from build123d import *

# Parameters (mm, degrees)
SKETCH_2_R                       = 1.75
EXTRUDE_1_DEPTH                  = 3
CUT_EXTRUDE_1_REACH              = 62.067
SKETCH_3_R                       = 13.5
EXTRUDE_START                    = -3
SKETCH_4_R                       = 3.75
SKETCH_4_R_2                     = 1.75
EXTRUDE_2_DEPTH                  = 3
FILLET_1_R                       = 1
PATTERN_CIRCULAR_1_COUNT         = 6
FILLET_1_OF_PATTERN_CIRCULAR_1_R = 1


with BuildPart() as part:
    # Sketch 2 → Extrude 1 (new body)
    # profile 1 of 5: a face of its own
    with BuildSketch(Plane(origin=(0, 0, 0), x_dir=(1, 0, 0), z_dir=(0, 1, 0))):
        with BuildLine():
            ThreePointArc((51.423130363, -9.332273137), (45.983390632, 4.986611908), (32.408442676, 12.08182334))
            ThreePointArc((32.408442676, 12.08182334), (21.996560251, 10.749395349), (13.44709691, 4.659293825))
            ThreePointArc((13.44709691, 4.659293825), (14.101694562, 1.915015852), (13.429705605, -0.82505541))
            ThreePointArc((13.429705605, -0.82505541), (11.883124263, -4.954311801), (11.357646636, -9.332273137))
            ThreePointArc((11.357646636, -9.332273137), (10.786787874, -12.531492943), (9.144672071, -15.335836498))
            ThreePointArc((9.144672071, -15.335836498), (13.315451151, -23.167946482), (20.286858748, -28.657647844))
            ThreePointArc((20.286858748, -28.657647844), (41.230232488, -27.655329089), (51.423130363, -9.332273137))
        make_face()
        with Locations(Location((16.434252877, -17.082273137, 0), (0, 0, 270))):
            Circle(SKETCH_2_R, mode=Mode.SUBTRACT)
        with Locations(Location((29.857646636, -24.832273137, 0), (0, 0, 270))):
            Circle(SKETCH_2_R, mode=Mode.SUBTRACT)
        with Locations(Location((43.281040395, -17.082273137, 0), (0, 0, 270))):
            Circle(SKETCH_2_R, mode=Mode.SUBTRACT)
        with Locations(Location((16.434252877, -1.582273137, 0), (0, 0, 270))):
            Circle(SKETCH_2_R, mode=Mode.SUBTRACT)
        with Locations(Location((43.281040395, -1.582273137, 0), (0, 0, 270))):
            Circle(SKETCH_2_R, mode=Mode.SUBTRACT)
        with Locations(Location((29.857646636, 6.167726863, 0), (0, 0, 270))):
            Circle(SKETCH_2_R, mode=Mode.SUBTRACT)
    # profile 2 of 5: a face of its own
    with BuildSketch(Plane(origin=(0, 0, 0), x_dir=(1, 0, 0), z_dir=(0, 1, 0))):
        with BuildLine():
            ThreePointArc((13.429705605, -0.82505541), (14.101694562, 1.915015852), (13.44709691, 4.659293825))
            ThreePointArc((13.44709691, 4.659293825), (8.774707488, -4.795780521), (9.144672071, -15.335836498))
            ThreePointArc((9.144672071, -15.335836498), (10.786787874, -12.531492943), (11.357646636, -9.332273137))
            ThreePointArc((11.357646636, -9.332273137), (11.883124263, -4.954311801), (13.429705605, -0.82505541))
        make_face()
    # profile 3 of 5: a face of its own
    with BuildSketch(Plane(origin=(0, 0, 0), x_dir=(1, 0, 0), z_dir=(0, 1, 0))):
        with BuildLine():
            ThreePointArc((-3.33566455, 16.339576043), (-3.689884424, 16.371156277), (-4.04535307, 16.381695363))
            Line((-4.04535307, 16.381695363), (-7.902002826, 16.381695363))
            ThreePointArc((-7.902002826, 16.381695363), (-11.154056436, 15.423931704), (-13.367877124, 12.856411137))
            ThreePointArc((-13.367877124, 12.856411137), (-13.731255095, 12.088797564), (-14.12049634, 11.333969504))
            ThreePointArc((-14.12049634, 11.333969504), (-14.757788596, 7.532855597), (-12.951275808, 4.128282218))
            ThreePointArc((-12.951275808, 4.128282218), (-8.656551428, -2.002025351), (-7.142353364, -9.332273137))
            ThreePointArc((-7.142353364, -9.332273137), (-5.751591288, -14.210272651), (-1.997514606, -17.62143179))
            ThreePointArc((-1.997514606, -17.62143179), (3.966394433, -18.393595151), (9.144672071, -15.335836498))
            ThreePointArc((9.144672071, -15.335836498), (8.774707488, -4.795780521), (13.44709691, 4.659293825))
            ThreePointArc((13.44709691, 4.659293825), (11.883867195, 6.59187417), (9.671521613, 7.725047131))
            ThreePointArc((9.671521613, 7.725047131), (4.722427963, 10.031982506), (0.837283213, 13.868794863))
            ThreePointArc((0.837283213, 13.868794863), (-0.988440561, 15.544571103), (-3.33566455, 16.339576043))
        make_face()
        with Locations(Location((2.107646636, -14.332273137, 0), (0, 0, 270))):
            Circle(SKETCH_2_R, mode=Mode.SUBTRACT)
        with Locations(Location((-2.222480383, -6.832273137, 0), (0, 0, 270))):
            Circle(SKETCH_2_R, mode=Mode.SUBTRACT)
        with Locations(Location((6.437773655, -6.832273137, 0), (0, 0, 270))):
            Circle(SKETCH_2_R, mode=Mode.SUBTRACT)
        with Locations(Location((8.10172473, 1.934042232, 0), (0, 0, 270))):
            Circle(SKETCH_2_R, mode=Mode.SUBTRACT)
        with Locations(Location((-7.902002826, 10.381695363, 0), (0, 0, 270))):
            Circle(SKETCH_2_R, mode=Mode.SUBTRACT)
    # profile 4 of 5: a face of its own
    with BuildSketch(Plane(origin=(0, 0, 0), x_dir=(1, 0, 0), z_dir=(0, 1, 0))):
        with BuildLine():
            Line((32.408442676, 12.08182334), (-3.33566455, 16.339576043))
            ThreePointArc((-3.33566455, 16.339576043), (-0.988440561, 15.544571103), (0.837283213, 13.868794863))
            ThreePointArc((0.837283213, 13.868794863), (4.722427963, 10.031982506), (9.671521613, 7.725047131))
            ThreePointArc((9.671521613, 7.725047131), (11.883867195, 6.59187417), (13.44709691, 4.659293825))
            ThreePointArc((13.44709691, 4.659293825), (21.996560251, 10.749395349), (32.408442676, 12.08182334))
        make_face()
    # profile 5 of 5: a face of its own
    with BuildSketch(Plane(origin=(0, 0, 0), x_dir=(1, 0, 0), z_dir=(0, 1, 0))):
        with BuildLine():
            Line((-1.997514606, -17.62143179), (20.286858748, -28.657647844))
            ThreePointArc((20.286858748, -28.657647844), (13.315451151, -23.167946482), (9.144672071, -15.335836498))
            ThreePointArc((9.144672071, -15.335836498), (3.966394433, -18.393595151), (-1.997514606, -17.62143179))
        make_face()
    extrude(amount=EXTRUDE_1_DEPTH)

    # Sketch 3 → Cut-Extrude 1 (cut, up to next)
    with BuildSketch(Plane(origin=(0, 3, 0), x_dir=(1, 0, 0), z_dir=(0, 1, 0)), mode=Mode.PRIVATE) as cut_extrude_1_sk1:
        with Locations(Location((29.857646636, -9.332273137, 0), (0, 0, 270))):
            Circle(SKETCH_3_R)
    cut_extrude_1_tool1 = extrude(cut_extrude_1_sk1.sketch, amount=-CUT_EXTRUDE_1_REACH, mode=Mode.PRIVATE) & part.part
    add(cut_extrude_1_tool1.solids().sort_by_distance((29.857647, 3, 9.332273))[0], mode=Mode.SUBTRACT)

    # Sketch 4 → Extrude 2 (add)
    with BuildSketch(Plane(origin=(0, 3, 0), x_dir=(1, 0, 0), z_dir=(0, 1, 0)).offset(EXTRUDE_START)):
        with Locations((29.857646636, 6.167726863)):
            Circle(SKETCH_4_R)
        with Locations(Location((29.857646636, 6.167726863, 0), (0, 0, 270))):
            Circle(SKETCH_4_R_2, mode=Mode.SUBTRACT)
    extrude_2 = extrude(amount=EXTRUDE_2_DEPTH)

    # Fillet 1
    fillet_1_edges = [part.edges().sort_by_distance(p)[0] for p in [
        (32.800222011, 1.5, -3.843130088),
        (26.915071261, 1.5, -3.843130088),
    ]]
    fillet(fillet_1_edges, radius=FILLET_1_R)

    # Pattern Circular 1: Extrude 2 ×6 about axis
    pattern_circular_1_axis = Axis((29.857646636, 0, 9.332273137), (0, 1, 0))
    for i in range(1, PATTERN_CIRCULAR_1_COUNT):
        add(extrude_2.rotate(pattern_circular_1_axis, i * 360 / PATTERN_CIRCULAR_1_COUNT))

    # Fillet 1 of Pattern Circular 1
    fillet_1_of_pattern_circular_1_edges = [part.edges().sort_by_distance(p)[0] for p in [
        (19.918700425, 1.5, 0.196226497),
        (16.97612505, 1.5, 5.292916552),
        (16.97612505, 1.5, 13.371629723),
        (19.918700425, 1.5, 18.468319778),
        (26.915071261, 1.5, 22.507676363),
        (32.800222011, 1.5, 22.507676363),
        (39.796592847, 1.5, 18.468319778),
        (42.739168222, 1.5, 13.371629723),
        (42.739168222, 1.5, 5.292916552),
        (39.796592847, 1.5, 0.196226497),
    ]]
    fillet(fillet_1_of_pattern_circular_1_edges, radius=FILLET_1_OF_PATTERN_CIRCULAR_1_R)


solid = part.part
Work out the finished part from the listing and answer in its coordinate system (mm). A direction names the side the tool comes from. Coordinates: 2 decimals unless noted, no trailing zeros. Write each loop counter-clockwise with the first axis right and the second up, starting at its lowest first coordinate (ties: lowest second). Pieces come first, ordered by that corner, then holes. Notation, with made-up numbers: M 79,30 L 111,30 A13 ccw 111,52 Z; hole C 8,18 d8. An arc over 180 degrees is marked long. Write item = value, one per line.
1. The part is cut by section A-A (z = -1). Determine the outline of the cut face in (x, y), then the cut area to 3 significant figures.
Solution:
outline = M -10.3,0 L 6.62,0 L 6.62,3 L -10.3,3 Z; M 9.58,0 L 21.17,0 L 21.17,3 L 9.58,3 Z; M 38.55,0 L 48.79,0 L 48.79,3 L 38.55,3 Z
area = 116 mm2
2. Determine the mould class of faces 1 (the face through (8.989, 1.479, 23.062)), 2 (the face through (40.054, 1.479, 15.173)), 3 (the face through (-6, 1, -16.382)) for opening direction Z: released by +Z, released by -Z, zero draft, split by the parting line, or undercut.
Solution:
face_1 = released by +Z
face_2 = undercut
face_3 = released by -Z
3. The part is cut by section C-C (z = 7.5). Determine the outline of the cut face in (x, y), then the cut area to 3 significant figures.
Solution:
outline = M -7.23,0 L -3.84,0 L -3.84,3 L -7.23,3 Z; M -0.6,0 L 4.82,0 L 4.82,3 L -0.6,3 Z; M 8.06,0 L 16.48,0 L 16.48,3 L 8.06,3 Z; M 43.23,0 L 51.35,0 L 51.35,3 L 43.23,3 Z
area = 76.1 mm2
4. A flat-ended cylindrical pin translates along its axis: pin 1 (1.5 mm diameter, centred on y = 2.5, z = 6.5, fed in from -X). Find the tip coordinate at first contact, or state that the pin passes through.
Solution:
pin_1 = -7.49
5. For faces 4 (the face through (-5.79, 1.48, 14.15)), 5 (the face through (19.662, 1.479, 3.492)), determine the directions among +Z, -Z, +X, -X, +Y, -Y from which every point of the face is accessible in a straight line to the end or side of a thin tool.
Solution:
face_4 = +Z, -X, +Y, -Y
face_5 = +Y, -Y
6. The part is cut by section B-B (x = 37). Determine the outline of the cut face in (y, z), then the cut area to 3 significant figures.
Solution:
outline = M 0,-11.02 L 3,-11.02 L 3,-2.12 L 0,-2.12 Z; M 0,20.79 L 3,20.79 L 3,29.68 L 0,29.68 Z
area = 53.4 mm2
7. The part is cut by section D-D (z = -10). Determine the outline of the cut face in (x, y), then the cut area to 3 significant figures.
Solution:
outline = M -14.64,0 L -9.61,0 L -9.61,3 L -14.64,3 Z; M -6.19,0 L 39.41,0 L 39.41,3 L -6.19,3 Z
area = 152 mm2
8. Straight lines are drawn through the part: line 1 (X direction, y = 2.65, z = 21.5); line 2 (X direction, y = 1.15, z = -3); line 3 (X direction, y = 2, z = 16.5). For each, find the intervals that lie inside material, in ascending order. Write a range as from..to.
Solution:
line_1 = 5.83..24.01, 28.14..31.58, 35.71..47.66
line_2 = -11.85..6.71, 9.49..24.37, 27.85..31.86, 35.35..47.55
line_3 = -3.74..14.78, 18.08..20.14, 39.58..41.63, 44.93..50.2
